Work out the finished part from the listing and answer in its coordinate system (mm). Coordinates: 2 decimals unless noted, no trailing zeros. Write each loop counter-clockwise with the first axis right and the second up, starting at its lowest first coordinate (ties: lowest second). Pieces come first, ordered by that corner, then holes. Notation, with made-up numbers: (83, 64.5) - (90, 64.5) arc R12 ccw to (90, 70.5) - close; hole circle Ø4 at (54.5, 29.5). An arc over 180 degrees is marked (long way). Use CSV: the item, a comma, the result in double quotes. Start each with the question number.
from build123d import *

# Parameters (mm, degrees)
F5_DEPTH      = 25
F7_DEPTH      = 343
F7_DEPTH_BACK = 50
F8_W          = 519.6738243103
F8_H          = 31.4134806395
F9_DEPTH      = 544


with BuildPart() as f5:
    # F4 (on 3pt) → F5 (new body)
    with BuildSketch(Plane(origin=(97.7491601024, 97.7491601024, 177.9939324181), x_dir=(0.9010441054, -0.2087794804, -0.3801718673), z_dir=(0.4337274722, 0.4337274722, 0.7897853884))):
        Polygon((-108.4843233732, 455.4515841965), (-108.4843233732, -137.3592433699), (468.1933296886, 0), align=None)
    extrude(amount=-F5_DEPTH)

    # F6 (on Top) → F7 (cut, two sides)
    with BuildSketch(Plane.XY) as f7_sk:
        Polygon((0, 577.9420137405), (-45, 577.9420137405), (-45, -45), (592.9301977158, -45), (592.9301977158, 0), (0, 0), align=None)
    extrude(amount=F7_DEPTH, mode=Mode.SUBTRACT)
    extrude(f7_sk.sketch, amount=-F7_DEPTH_BACK, mode=Mode.SUBTRACT)

    # F8 (on Front) → F9 (cut)
    with BuildSketch(Plane.XZ):
        with Locations((259.8369121552, -15.7067403197)):
            Rectangle(F8_W, F8_H)
    extrude(amount=-F9_DEPTH, mode=Mode.SUBTRACT)


solid = f5.part
Item 1: Straight lines are drawn through the part: probe 1 along Z at (x, y) = (232, 73.5); probe 2 along Z at (x, y) = (329, 151.5); probe 3 along X at (y, z) = (71, 94) (3 decimals). For each, find the intervals that lie inside material, in ascending order. Write a range as [from, to].
Item 2: A cutting plane is placed at A-A (y = 447). Determine the outline of the cut face in (x, z).
Item 3: Each of these flat-tipped pins is pushed along its axis until it touches: pin 1 (3 mm diameter, centred on x = 181, y = 295, fed in from +Z); pin 2 (3 mm diameter, centred on x = 77.5, y = 97, fed in from -Z); pin 3 (12 mm diameter, centred on x = 216, y = 105.5, fed in from +Z). Where does it stop, or does it pass through?
Item 4: Determine the mould class of faces 1 (the face through (259, 259, 0)), 2 (the face through (140.7, 173.11, 113.02)), 3 (the face through (125.092, 153.905, 100.485)) for opening direction Y: +Y half, -Y half, draft (parallel to the pull), parting line (faces both ways), or undercut.
Item 5: A cutting plane is placed at B-B (z = 202). Determine the outline of the cut face in (x, y).
Calculated:
1,probe 1,"z = [85.93, 117.58]"
1,probe 2,"z = [0, 21.48]"
1,probe 3,"x = [219.805, 277.445]"
2,outline,"(0, 8.22) - (14.97, 0) - (72.61, 0) - (0, 39.88) - close"
3,pin 1,"stops at z = 25.12"
3,pin 2,"stops at z = 156.71"
3,pin 3,"stops at z = 113.46"
4,face 1,"draft"
4,face 2,"+Y half"
4,face 3,"-Y half"
5,outline,"(0, 94.15) - (94.15, 0) - (151.79, 0) - (0, 151.79) - close"
